The model under review builds one solid part; all positions refer to its coordinate system, in mm. A direction names the side the tool comes from. Give positions to 0.01 mm unless a question says otherwise; leave off trailing zeros. Loops run counter-clockwise (first coordinate to the right, second up) from the corner with the lowest first, then second, coordinate; pieces in that order, holes last. Notation, with made-up numbers: M 46.25,56 L 100.25,56 A17 cw 100.25,60 Z; hole C 25,52 d8. An arc over 180 degrees is marked long. Put each result on its own line as item: value. Start each with the question number.
from build123d import *

# Parameters (mm, degrees)
F2_DEPTH = 25.4
F3_DEPTH = 25.4


with BuildPart() as f2:
    # F0 (on Right) → F2 (new body)
    with BuildSketch(Plane.YZ):
        with BuildLine():
            ThreePointArc((-5.555995, -18.155882), (-17.114845, -3.483872), (-11.34728, 14.281546))
            Line((-11.34728, 14.281546), (-90.925781, 7.443868))
            ThreePointArc((-90.925781, 7.443868), (-88.017793, 4.215689), (-86.966366, 0))
            ThreePointArc((-86.966366, 0), (-87.125503, -1.682815), (-87.597275, -3.305968))
            Line((-87.597275, -3.305968), (-5.555995, -18.155882))
        make_face()
        with BuildLine():
            ThreePointArc((-86.966366, 0), (-88.017793, 4.215689), (-90.925781, 7.443868))
            ThreePointArc((-90.925781, 7.443868), (-104.518898, -2.655239), (-87.597275, -3.305968))
            ThreePointArc((-87.597275, -3.305968), (-87.125503, -1.682815), (-86.966366, 0))
        make_face()
        with BuildLine():
            ThreePointArc((-5.555995, -18.155882), (13.243766, -16.591974), (22.220583, 0))
            ThreePointArc((22.220583, 0), (10.158773, 18.239819), (-11.34728, 14.281546))
            ThreePointArc((-11.34728, 14.281546), (-17.114845, -3.483872), (-5.555995, -18.155882))
        make_face()
    extrude(amount=F2_DEPTH)

    # F0 (on Right) → F3 (join)
    with BuildSketch(Plane.YZ):
        with BuildLine():
            ThreePointArc((-5.555995, -18.155882), (13.243766, -16.591974), (22.220583, 0))
            ThreePointArc((22.220583, 0), (10.158773, 18.239819), (-11.34728, 14.281546))
            ThreePointArc((-11.34728, 14.281546), (-17.114845, -3.483872), (-5.555995, -18.155882))
        make_face()
        with BuildLine():
            ThreePointArc((-5.555995, -18.155882), (-17.114845, -3.483872), (-11.34728, 14.281546))
            Line((-11.34728, 14.281546), (-90.925781, 7.443868))
            ThreePointArc((-90.925781, 7.443868), (-88.017793, 4.215689), (-86.966366, 0))
            ThreePointArc((-86.966366, 0), (-87.125503, -1.682815), (-87.597275, -3.305968))
            Line((-87.597275, -3.305968), (-5.555995, -18.155882))
        make_face()
        with BuildLine():
            ThreePointArc((-86.966366, 0), (-88.017793, 4.215689), (-90.925781, 7.443868))
            ThreePointArc((-90.925781, 7.443868), (-104.518898, -2.655239), (-87.597275, -3.305968))
            ThreePointArc((-87.597275, -3.305968), (-87.125503, -1.682815), (-86.966366, 0))
        make_face()
    extrude(amount=F3_DEPTH)


solid = f2.part
(1) Draft analysis for pull direction Y (two halves, no side actions). For faces 3 (the flat face through (0, -28, 0)), 4 (the flat face through (12.52, -50.58, 10.91)), state which applies: +Y half, -Y half, draft (parallel to the pull), parting line (faces both ways), or undercut.
(2) We need section B-B, the plane y = -29.5. Write out the cut boundary in (x, z).
(3) For faces 1 (the flat face through (12.522, -47.151, -10.627)), 2 (the cylindrical face through (12.522, -104.605, -2.358)), list the 3-axis set-ups (+Z, -Z, +X, -X, +Y, -Y) from which the entire face can be reached by the end or side of a thin tool; tool diameter is ignored.
(4) We need section C-C, the plane z = -11. Write out the cut boundary in (x, y).
(5) We need section A-A, the plane x = 13.5. Write out the cut boundary in (y, z).
(6) To check wall thickness, follow L1, parallel to Z at x = 1.25, y = -96.5; L2, parallel to Y at x = 4.5, z = -3; L3, parallel to Z at x = 21.5, y = -89.5. State the ranges of each line that lie inside material, in increasing order. Write a range as [from, to].
(7) Insertion check: pin 1 (12 mm diameter, centred on x = 15, y = -59.5, fed in from +Z); pin 2 (6 mm diameter, centred on x = 10, y = -63, fed in from +Z); pin 3 (8 mm diameter, centred on x = 10.5, y = -21, fed in from +Z). Each pin has a flat end and moves straight along its axis. Give the tip position at first contact, or say it passes through.
Check sheet entries:
1. face 3: draft
1. face 4: undercut
2. outline: M 0,-13.82 L 25.4,-13.82 L 25.4,12.72 L 0,12.72 Z
3. face 1: -Z, +X, -X
3. face 2: +X, -X
4. outline: M 0,-45.09 L 25.4,-45.09 L 25.4,18.89 L 0,18.89 Z
5. outline: M -90.93,7.44 A8.98 ccw long -87.6,-3.31 L -5.56,-18.16 A19.82 ccw long -11.35,14.28 Z
6. L1: z = [-8.96, 8.96]
6. L2: y = [-104.4, 21.99]
6. L3: z = [-6.25, 7.57]
7. pin 1: stops at z = 10.66
7. pin 2: stops at z = 10.1
7. pin 3: stops at z = 13.8
